Geometry check sheet. Reference: drawing and pictorial views, mm from the part's lowest x, y, z. A direction names the side the tool comes from. Coordinates: 2 decimals unless noted, no trailing zeros. Loops run counter-clockwise (first coordinate to the right, second up) from the corner with the lowest first, then second, coordinate; pieces in that order, holes last. Notation, with made-up numbers: (-24, 50) -> (-7, 50) arc R22 cw to (-7, 85) -> close; hole circle Ø6 at (38.25, 39.5). An arc over 180 degrees is marked (long way). Use CSV: the item, a comma, the result in double quotes.
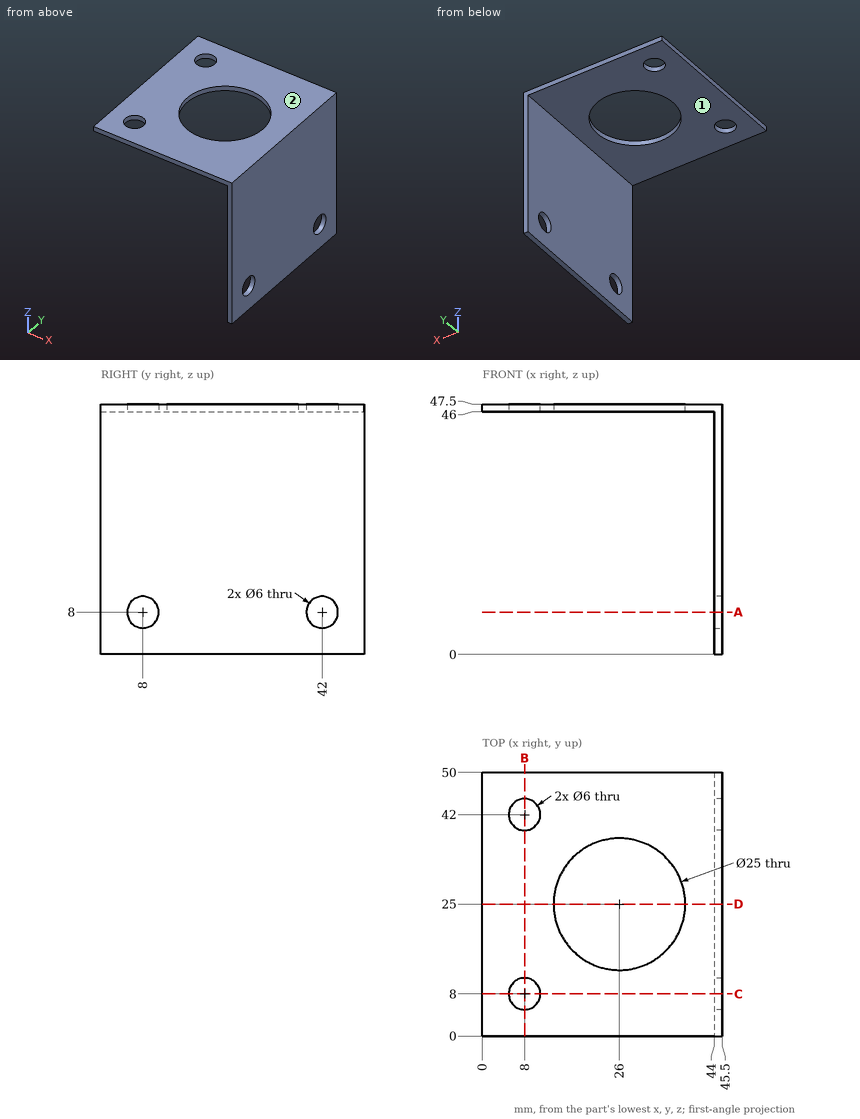
1) Cross-section at D-D on y = 25. Record the boundary of the cut face in (x, z), and give its area (4 significant figures).
Answer below:
outline,"(0, 46) -> (13.5, 46) -> (13.5, 47.5) -> (0, 47.5) -> close; (38.5, 46) -> (44, 46) -> (44, 0) -> (45.5, 0) -> (45.5, 47.5) -> (38.5, 47.5) -> close"
area,"99.75 mm²"
2) Cross-section at B-B on x = 8. Record the boundary of the cut face in (y, z).
Answer below:
outline,"(0, 46) -> (5, 46) -> (5, 47.5) -> (0, 47.5) -> close; (11, 46) -> (39, 46) -> (39, 47.5) -> (11, 47.5) -> close; (45, 46) -> (50, 46) -> (50, 47.5) -> (45, 47.5) -> close"
3) Go/stop test with flat-tipped pins: pin 1 Ø14 at (y, z) = (32, 29) entering from -X; pin 2 Ø5.5 at (y, z) = (8, 8) entering from -X; pin 3 Ø22 at (x, y) = (22, 19.5) entering from -Z. Record where each tip stops, or that it passes through.
Answer below:
pin 1,"stops at x = 44"
pin 2,"passes through"
pin 3,"stops at z = 46"
4) Access from +Z, -Z, +X, -X, +Y, -Y to the whole of each face (thin tool, end or side, straight path). Record for the marked faces 1 and 2.
Answer below:
face 1,"-Z, -X, +Y, -Y"
face 2,"+Z, +X, -X, +Y, -Y"
5) Cross-section at A-A on z = 8. Record the boundary of the cut face in (x, y), and give its area (3 significant figures).
Answer below:
outline,"(44, 0) -> (45.5, 0) -> (45.5, 5) -> (44, 5) -> close; (44, 11) -> (45.5, 11) -> (45.5, 39) -> (44, 39) -> close; (44, 45) -> (45.5, 45) -> (45.5, 50) -> (44, 50) -> close"
area,"57.0 mm²"
6) Cross-section at C-C on y = 8. Record the boundary of the cut face in (x, z).
Answer below:
outline,"(0, 46) -> (5, 46) -> (5, 47.5) -> (0, 47.5) -> close; (11, 46) -> (44, 46) -> (44, 11) -> (45.5, 11) -> (45.5, 47.5) -> (11, 47.5) -> close; (44, 0) -> (45.5, 0) -> (45.5, 5) -> (44, 5) -> close"
7) Thickness scan on line 1 along Y through (x, z) = (45, 8); line 2 along Z through (x, y) = (2, 12.5); line 3 along X through (y, z) = (41.5, 15). Record the ranges inside material, lowest first. Write a range as from..to.
Answer below:
line 1,"y = 0..5, 11..39, 45..50"
line 2,"z = 46..47.5"
line 3,"x = 44..45.5"
